```python
from build123d import *

# Parameters (mm, degrees)
F3_D      = 13.4874
F6_D      = 6.35
F6_DEPTH  = 6.35
F6_TIP    = 1.9077324654
F8_D      = 6.35
F8_DEPTH  = 6.35
F8_TIP    = 1.9077324654
F10_D     = 5.1054
F10_DEPTH = 19.05
F10_TIP   = 1.5338169022


with BuildPart() as f1:
    # F0 (on Front) → F1 (revolve)
    with BuildSketch(Plane.XZ):
        Polygon((0, 52.9336), (0, 0), (12.7, 0), (12.7, 30.1625), (25.4, 30.1625), (25.4, 36.2712), (22.86, 36.2712), (22.86, 50.5587), (22.225, 50.5587), (22.225, 52.9336), align=None)
    revolve(axis=Axis((0, 0, 26.4668), (0, 0, 1)))

    # F3 (through all)
    with Locations(Plane(origin=(0, 0, 0), x_dir=(1, 0, 0), z_dir=(0, 0, -1))):
        with Locations((0, 0)):
            Hole(F3_D / 2)

    # F6
    with Locations(Plane.XY.offset(52.9336)):
        with Locations((-14.1732, 7.8232), (14.1732, 7.8232)):
            Hole(F6_D / 2, depth=F6_DEPTH)
            with Locations((0, 0, -(F6_DEPTH + F6_TIP / 2))):  # 118° drill point
                Cone(0, F6_D / 2, F6_TIP, mode=Mode.SUBTRACT)

    # F8
    with Locations(Plane.XY.offset(52.9336)):
        with Locations((-14.9352, -7.8232), (14.1732, -7.8232)):
            Hole(F8_D / 2, depth=F8_DEPTH)
            with Locations((0, 0, -(F8_DEPTH + F8_TIP / 2))):  # 118° drill point
                Cone(0, F8_D / 2, F8_TIP, mode=Mode.SUBTRACT)

    # F10
    with Locations(Plane.XY.offset(52.9336)):
        with Locations((0, -14.2875), (0, 14.2875)):
            Hole(F10_D / 2, depth=F10_DEPTH)
            with Locations((0, 0, -(F10_DEPTH + F10_TIP / 2))):  # 118° drill point
                Cone(0, F10_D / 2, F10_TIP, mode=Mode.SUBTRACT)


solid = f1.part
```
The listing builds one solid part. Answer for the finished solid, in the listing's coordinates (mm). A direction names the side the tool comes from. Coordinates: 2 decimals unless noted, no trailing zeros. Write each loop counter-clockwise with the first axis right and the second up, starting at its lowest first coordinate (ties: lowest second). Pieces come first, ordered by that corner, then holes. Notation, with made-up numbers: (17, 83.5) - (38, 83.5) arc R21 cw to (38, 106.5) - close; hole circle Ø10 at (-14.75, 52.25). An arc over 180 degrees is marked (long way). Return JSON: item names as keys, results as strings. Group by question number.
1. A cutting plane is placed at D-D, the plane y = -20. Determine the outline of the cut face in (x, z).
2. Straight lines are drawn through the part: L1, parallel to Y at x = 0, z = 39.5; L2, parallel to Z at x = 10, y = -12.5; L3, parallel to Y at x = -3, z = 35. For each, find the intervals that lie inside material, in ascending order.
3. A cutting plane is placed at C-C, the plane z = 12. Determine the outline of the cut face in (x, y), plus the area to 3 significant figures.
4. A cutting plane is placed at A-A, the plane y = 0. Determine the outline of the cut face in (x, z) (1 decimal), plus the area to 3 significant figures.
5. A cutting plane is placed at B-B, the plane z = 45.5. Determine the outline of the cut face in (x, y), plus the area to 3 significant figures.
6. Which of the six approach directions +Z, -Z, +X, -X, +Y, -Y give full straight-line access (tool end or side, diameter ignored) to faces 1 (the flat face through (-19, 12, 50.559)), 2 (the flat face through (-5, -5, 0)), 3 (the flat face through (-5, 12, 30.162))?
7. Given pin 1 (2 mm diameter, centred on y = -13, z = 38.5, fed in from -X); pin 2 (7.5 mm diameter, centred on x = -14.94, y = -7.82, fed in from -Z); pin 3 (1.5 mm diameter, centred on x = -3, z = 35.5, fed in from -Y), each flat-ended and moving along its own axis, determine where each tip first touches the part or whether it passes through.
8. Determine the mould class of faces 4 (the cylindrical face through (-13.76, 10.97, 49.71)), 5 (the cylindrical face through (-5.506, -24.796, 33.26)), 6 (the flat face through (-5, -5, 52.934)), 7 (the conical face through (-0.058, -13.848, 32.616)) for opening direction Y: released by +Y, released by -Y, zero draft, split by the parting line, or undercut.
Ans:
{
 "1": {"outline": "(-15.66, 30.16) - (15.66, 30.16) - (15.66, 36.27) - (11.07, 36.27) - (11.07, 50.56) - (9.69, 50.56) - (9.69, 52.93) - (-9.69, 52.93) - (-9.69, 50.56) - (-11.07, 50.56) - (-11.07, 36.27) - (-15.66, 36.27) - close"},
 "2": {"L1": "-22.86 to -16.84, -11.73 to -6.74, 6.74 to 11.73, 16.84 to 22.86", "L2": "30.16 to 52.93", "L3": "-25.22 to -6.04, 6.04 to 25.22"},
 "3": {"outline": "circle Ø25.4 at (0, 0); hole circle Ø13.49 at (0, 0)", "area": "364 mm²"},
 "4": {"outline": "(-25.4, 30.2) - (-12.7, 30.2) - (-12.7, 0) - (-6.7, 0) - (-6.7, 52.9) - (-22.2, 52.9) - (-22.2, 50.6) - (-22.9, 50.6) - (-22.9, 36.3) - (-25.4, 36.3) - close; (6.7, 0) - (12.7, 0) - (12.7, 30.2) - (25.4, 30.2) - (25.4, 36.3) - (22.9, 36.3) - (22.9, 50.6) - (22.2, 50.6) - (22.2, 52.9) - (6.7, 52.9) - close", "area": "1,120 mm²"},
 "5": {"outline": "circle Ø45.72 at (0, 0); hole circle Ø2.74 at (-14.94, -7.82); hole circle Ø2.74 at (-14.17, 7.82); hole circle Ø13.49 at (0, 0); hole circle Ø5.11 at (0, -14.29); hole circle Ø5.11 at (0, 14.29); hole circle Ø2.74 at (14.17, -7.82); hole circle Ø2.74 at (14.17, 7.82)", "area": "1,430 mm²"},
 "6": {"face 1": "+Z", "face 2": "-Z, +X, -X, +Y, -Y", "face 3": "-Z"},
 "7": {"pin 1": "x = -19.46", "pin 2": "z = 30.16", "pin 3": "y = -25.3"},
 "8": {"face 4": "undercut", "face 5": "split by the parting line", "face 6": "zero draft", "face 7": "undercut"}
}
